from build123d import *

# Parameters (mm, degrees)
SKETCH_1_W          = 99
SKETCH_1_H          = 19
EXTRUDE_1_DEPTH     = 19.6
SKETCH_3_W          = 41
SKETCH_3_H          = 19.6
CUT_EXTRUDE_1_DEPTH = 9.8
SKETCH_6_W          = 20
SKETCH_6_H          = 19.6
CUT_EXTRUDE_2_DEPTH = 15.5
SHELL_2_T           = -2
SKETCH_7_W          = 99
SKETCH_7_H          = 19.6
EXTRUDE_3_DEPTH     = 0.5
SKETCH_21_W         = 20
SKETCH_21_H         = 9.8
CUT_EXTRUDE_3_DEPTH = 6.5


with BuildPart() as part:
    # 草圖1 → 填料-伸長1 (new body)
    with BuildSketch(Plane.XY):
        Rectangle(SKETCH_1_W, SKETCH_1_H)
    extrude(amount=EXTRUDE_1_DEPTH)

    # 草圖3 → 除料-伸長1 (cut)
    with BuildSketch(Plane(origin=(0, 9.5, 0), x_dir=(1, 0, 0), z_dir=(0, 1, 0))):
        with Locations((0, -9.8)):
            Rectangle(SKETCH_3_W, SKETCH_3_H)
    extrude(amount=-CUT_EXTRUDE_1_DEPTH, mode=Mode.SUBTRACT)

    # 草圖6 → 除料-伸長2 (cut)
    with BuildSketch(Plane(origin=(0, -0.3, 0), x_dir=(1, 0, 0), z_dir=(0, 1, 0))):
        Rectangle(SKETCH_6_W, SKETCH_6_H)
    extrude(amount=-CUT_EXTRUDE_2_DEPTH, mode=Mode.SUBTRACT)

    # 薄殼2
    shell_2_openings = [part.faces().sort_by_distance(p)[0] for p in [
        (0, -9.5, 10.350561798),
    ]]
    offset(amount=SHELL_2_T, openings=shell_2_openings, kind=Kind.INTERSECTION)

    # 草圖7 → 填料-伸長3 (add)
    with BuildSketch(Plane.XZ.offset(9.5)):
        with Locations((0, 9.8)):
            Rectangle(SKETCH_7_W, SKETCH_7_H)
    extrude(amount=-EXTRUDE_3_DEPTH)

    # 草圖21 → 除料-伸長3 (cut)
    with BuildSketch(Plane(origin=(0, -9, 0), x_dir=(1, 0, 0), z_dir=(0, 1, 0))):
        with Locations((0, -4.9)):
            Rectangle(SKETCH_21_W, SKETCH_21_H)
    extrude(amount=-CUT_EXTRUDE_3_DEPTH, mode=Mode.SUBTRACT)


solid = part.part
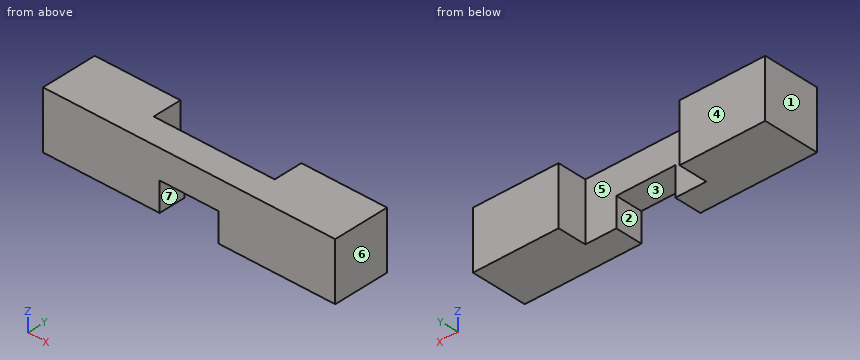
Could you check a few things on this model? Use its own coordinates, in mm. Face numbers are marked on the shaded views. A direction names the side the tool comes from. Round coordinates to 2 decimals unless told otherwise and drop trailing zeros. Loops run counter-clockwise (first coordinate to the right, second up) from the corner with the lowest first, then second, coordinate; pieces in that order, holes last. Notation, with made-up numbers: (-19, -24) - (17, -24) arc R31 ccw to (17, 0) - close; hole circle Ø7 at (66.5, 70). An arc over 180 degrees is marked (long way). Write item = value, one per line.
1) On a 3-axis mill with a long thin cutter (end or side, diameter ignored), from which of +Z, -Z, +X, -X, +Y, -Y can I reach the whole of each face in a straight line? I mean the marked faces 5, 6 and 7. Say none if no direction works.
Computed:
face_5 = +Z, -Z, +Y
face_6 = +Z, -Z, +X, +Y, -Y
face_7 = -Z, +Y, -Y
2) Imagine slicing it at C-C (x = -11). Please give me the cut outline in (y, z), and give its area (3 significant figures).
Computed:
outline = (-9.5, 0) - (-0.3, 0) - (-0.3, 19.6) - (-9.5, 19.6) - close; hole (-9, 11.8) - (-2.3, 11.8) - (-2.3, 17.6) - (-9, 17.6) - close
area = 141 mm2
3) Imagine slicing it at D-D (z = 16.25). Please give me the cut outline in (x, y), and give its area (3 significant figures).
Computed:
outline = (-49.5, -9.5) - (49.5, -9.5) - (49.5, 9.5) - (20.5, 9.5) - (20.5, -0.3) - (-20.5, -0.3) - (-20.5, 9.5) - (-49.5, 9.5) - close; hole (-47.5, -9) - (47.5, -9) - (47.5, 7.5) - (22.5, 7.5) - (22.5, -2.3) - (-22.5, -2.3) - (-22.5, 7.5) - (-47.5, 7.5) - close
area = 353 mm2
4) If we mould it in two halves opening along X, with no side actions, what happens to the marked faces 1, 2, 3 and 4? For each: pulls with the +X half, pulls with the -X half, needs draft (parallel to the pull), parting line crosses it, or undercut.
Computed:
face_1 = pulls with the -X half
face_2 = undercut
face_3 = undercut
face_4 = needs draft
5) I'm going to push a flat-ended pin straight in: P1, Ø7.5, axis at x = 3, y = -3.5, coming from the -Z side. Where does the tip first touch, or does it pass through?
Computed:
P1 = 9.8
6) Imagine slicing it at A-A (z = 6.75). Please give me the cut outline in (x, y).
Computed:
outline = (-49.5, -9.5) - (-10, -9.5) - (-10, -0.3) - (-20.5, -0.3) - (-20.5, 9.5) - (-49.5, 9.5) - close; (10, -9.5) - (49.5, -9.5) - (49.5, 9.5) - (20.5, 9.5) - (20.5, -0.3) - (10, -0.3) - close; hole (-47.5, -9) - (-12, -9) - (-12, -2.3) - (-22.5, -2.3) - (-22.5, 7.5) - (-47.5, 7.5) - close; hole (12, -9) - (47.5, -9) - (47.5, 7.5) - (22.5, 7.5) - (22.5, -2.3) - (12, -2.3) - close
7) I need wall thicknesses on line 1 along X through (y, z) = (-1.75, 5.75); line 2 along X through (y, z) = (2, 11.5); line 3 along X through (y, z) = (-2, 12.75). Which ranges of each line are inside material? Lowest first, please. Write a range as from..to.
Computed:
line_1 = -49.5..-47.5, -22.5..-10, 10..22.5, 47.5..49.5
line_2 = -49.5..-47.5, -22.5..-20.5, 20.5..22.5, 47.5..49.5
line_3 = -49.5..-47.5, -22.5..22.5, 47.5..49.5
8) Imagine slicing it at B-B (y = 4.5). Please give me the cut outline in (x, z).
Computed:
outline = (-49.5, 0) - (-20.5, 0) - (-20.5, 19.6) - (-49.5, 19.6) - close; (20.5, 0) - (49.5, 0) - (49.5, 19.6) - (20.5, 19.6) - close; hole (-47.5, 2) - (-22.5, 2) - (-22.5, 17.6) - (-47.5, 17.6) - close; hole (22.5, 2) - (47.5, 2) - (47.5, 17.6) - (22.5, 17.6) - close
